from build123d import *

# Parameters (mm, degrees)
F1_DEPTH = 19.05
F3_DEPTH = 134.874


with BuildPart() as f1:
    # F0 (on Top) → F1 (new body)
    with BuildSketch(Plane.XY):
        with BuildLine():
            Line((-12.7, 0), (0, 0))
            Line((0, 0), (0, 12.7))
            ThreePointArc((0, 12.7), (-8.9802561211, 8.9802561211), (-12.7, 0))
        make_face()
        with BuildLine():
            Line((0, 12.7), (0, 0))
            Line((0, 0), (12.7, 0))
            ThreePointArc((12.7, 0), (8.9802561211, 8.9802561211), (0, 12.7))
        make_face()
        with BuildLine():
            Line((12.7, 0), (0, 0))
            Line((0, 0), (0, -12.7))
            ThreePointArc((0, -12.7), (8.9802561211, -8.9802561211), (12.7, 0))
        make_face()
        with BuildLine():
            Line((0, -12.7), (0, 0))
            Line((0, 0), (-12.7, 0))
            ThreePointArc((-12.7, 0), (-8.9802561211, -8.9802561211), (0, -12.7))
        make_face()
    extrude(amount=F1_DEPTH)

    # F2 (on face) → F3 (cut)
    with BuildSketch(Plane.XY.offset(19.05)):
        with BuildLine():
            Line((-1.778, 0), (0, 0))
            Line((0, 0), (0, 1.778))
            ThreePointArc((0, 1.778), (-1.2572358569, 1.2572358569), (-1.778, 0))
        make_face()
        with BuildLine():
            Line((0, 1.778), (0, 0))
            Line((0, 0), (1.778, 0))
            ThreePointArc((1.778, 0), (1.2572358569, 1.2572358569), (0, 1.778))
        make_face()
        with BuildLine():
            Line((1.778, 0), (0, 0))
            Line((0, 0), (0, -1.778))
            ThreePointArc((0, -1.778), (1.2572358569, -1.2572358569), (1.778, 0))
        make_face()
        with BuildLine():
            Line((0, -1.778), (0, 0))
            Line((0, 0), (-1.778, 0))
            ThreePointArc((-1.778, 0), (-1.2572358569, -1.2572358569), (0, -1.778))
        make_face()
    extrude(amount=-F3_DEPTH, mode=Mode.SUBTRACT)


solid = f1.part
Model file for the job. Use its own axes, mm. Give positions to 0.01 mm unless a question says otherwise; leave off trailing zeros. Write each loop counter-clockwise with the first axis right and the second up, starting at its lowest first coordinate (ties: lowest second). Pieces come first, ordered by that corner, then holes. Notation, with made-up numbers: M 21.5,44 L 49.5,44 A21 ccw 49.5,69 Z; hole C 16.25,-38 d4. An arc over 180 degrees is marked long. One line per item, written item: value. Start each with the question number.
Q1. Probe probe 1 along X at (y, z) = (-0.75, 14); probe 2 along Y at (x, z) = (4.75, 1); probe 3 along X at (y, z) = (-8.5, 12.25). List the from-to ranges inside material, lowest first. Write a range as [from, to].
Q2. Saw through at B-B, the plane x = 9.25. Write the cut outline in (y, z), plus the area to 3 significant figures.
Q3. Saw through at C-C, the plane y = 10.5. Write the cut outline in (x, z).
Q4. Saw through at A-A, the plane z = 8.25. Write the cut outline in (x, y), plus the area to 3 significant figures.
Q5. Drop flat-ended pins along their axis: pin 1 Ø12 at (x, y) = (-4, 0.5) entering from -Z; pin 2 Ø2 at (x, z) = (-5, 15) entering from +Y; pin 3 Ø8 at (y, z) = (8, 9) entering from +X; pin 4 Ø2 at (x, z) = (-5.5, 14) entering from -Y. Give the stop position or say it passes through.
Output values:
1. probe 1: x = [-12.68, -1.61], [1.61, 12.68]
1. probe 2: y = [-11.78, 11.78]
1. probe 3: x = [-9.44, 9.44]
2. outline: M -8.7,0 L 8.7,0 L 8.7,19.05 L -8.7,19.05 Z
2. area: 332 mm²
3. outline: M -7.14,0 L 7.14,0 L 7.14,19.05 L -7.14,19.05 Z
4. outline: C 0,0 d25.4; hole C 0,0 d3.56
4. area: 497 mm²
5. pin 1: stops at z = 0
5. pin 2: stops at y = 12.05
5. pin 3: stops at x = 12.05
5. pin 4: stops at y = -11.88
